Source: CAD feature listing. Evaluate the final solid. Frame: model axes, mm. A direction names the side the tool comes from. Give positions to 0.01 mm unless a question says otherwise; leave off trailing zeros. Order: outer loops, then holes, each group sorted by start corner. A loop starts at its lowest first (then second) coordinate and runs counter-clockwise, first axis right, second up.
Autodesk Fusion 360 part; units mm, degrees
sketch "Boceto1" plane through (0, 0, 0) normal (0, 1, 0) x (1, 0, 0)
  line L0 (0, -3) -> (0, -6)
  line L1 (0, -6) -> (30, -6)
  line L2 (30, -6) -> (30, -3.5)
  line L3 (30, -3.5) -> (9, -3.5)
  line L4 (9, -3.5) -> (8.4641, -1.5)
  line L5 (8.4641, -1.5) -> (3.5, -1.5)
  line L6 (3.5, -1.5) -> (3.5, -3)
  line L7 (0, -3) -> (3.5, -3)
  line L8 (0, 0) -> (32.7199, 0) construction
  dimension "d2" = 21
  dimension "d3" = 3.5
  dimension "d4" = 30
  dimension "d8" = 3
  dimension "d9" = 1.5
  dimension "d10" = 6
  dimension "d11" = 3.5
  dimension "d13" = 75
revolve "Revolución1" add sketch "Boceto1" angle 360 about axis through (0, 0, 0) along (1, 0, 0)
sketch "Boceto2" plane through (0, 0, 0) normal (0, 0, 1) x (1, 0, 0)
  circle A0 centre (24, 0) radius 1
  circle A1 centre (17, 0) radius 1
  circle A2 centre (2.5, 0) radius 1
  point P0 (30, 0)
  dimension "d15" = 2.5
  dimension "d16" = 2
  dimension "d17" = 2
  dimension "d18" = 2
  dimension "d19" = 6
  dimension "d20" = 13
extrude "Extruir1" cut sketch "Boceto2" along normal mid plane 14
1) Pin query (flat end, axial travel): pin 1 (3 mm diameter, centred on x = 2.5, y = 0, fed in from +Z); pin 2 (1.2 mm diameter, centred on x = 17, y = 0, fed in from +Z); pin 3 (1 mm diameter, centred on x = 5, z = 1.5, fed in from -Y); pin 4 (3.5 mm diameter, centred on y = 0, z = 0, fed in from +X). Return the tip coordinate at first contact, or that it passes through.
Report:
pin 1: stops at z = 6
pin 2: passes through
pin 3: stops at y = -5.92
pin 4: stops at x = 8.53
2) Section query C-C, the plane x = 5.5. Return the cut outline in (y, z).
Report:
outline: circle Ø12 at (0, 0); hole circle Ø3 at (0, 0)
3) Draft query along Z for faces 3 (the cylindrical face through (19.35, 1.05, 3.34)), 4 (the flat face through (3.5, 1.3, 1.3)), 5 (the cylindrical face through (17, 1, 5)), 6 (the cylindrical face through (15.21, -1.802, 5.723)). Return one class per face: +Z half, -Z half, draft (parallel to the pull), parting line (faces both ways), or undercut.
Report:
face 3: undercut
face 4: undercut
face 5: draft
face 6: parting line
4) Section query A-A, the plane z = 0. Return the cut outline in (x, y), and give its area (3 significant figures).
Report:
outline: (0, -6) - (30, -6) - (30, -3.5) - (9, -3.5) - (8.46, -1.5) - (3.5, -1.5) - (3.5, -3) - (0, -3) - close; (0, 3) - (3.5, 3) - (3.5, 1.5) - (8.46, 1.5) - (9, 3.5) - (30, 3.5) - (30, 6) - (0, 6) - close
area: 174 mm2
5) Reachability of faces 1 (the flat face through (0, 1, -3)), 2 (the cylindrical face through (1.77, 1.15, 2.77)) from +Z, -Z, +X, -X, +Y, -Y: full face, straight path, thin tool, end or side. Return the list, or none.
Report:
face 1: +Z, -Z, -X, +Y, -Y
face 2: -X
6) Material intervals for L1, parallel to X at y = 0, z = -5.1; L2, parallel to Z at x = 5, y = 0; L3, parallel to Z at x = 27, y = 0, sorted ascending.
Report:
L1: x = 0 to 1.5, 3.5 to 16, 18 to 23, 25 to 30
L2: z = -6 to -1.5, 1.5 to 6
L3: z = -6 to -3.5, 3.5 to 6
7) Section query B-B, the plane x = 17. Return the cut outline in (y, z), and give its area (3 significant figures).
Report:
outline: (-1, -5.92) - (-1, -3.35) arc R3.5 cw to (-1, 3.35) - (-1, 5.92) arc R6 ccw to start; (1, -5.92) arc R6 ccw to (1, 5.92) - (1, 3.35) arc R3.5 cw to (1, -3.35) - close
area: 64.5 mm2
8) Section query D-D, the plane y = -5. Return the cut outline in (x, z), and give its area (3 significant figures).
Report:
outline: (0, -3.32) - (30, -3.32) - (30, 3.32) - (0, 3.32) - close
area: 199 mm2
